from build123d import *

# Parameters (mm, degrees)
BOSS_EXTRUDE1_DEPTH = 165
SKETCH2_R           = 2.5
CUT_EXTRUDE1_DEPTH  = 167.021082999
SKETCH3_R           = 2.5
CUT_EXTRUDE2_DEPTH  = 167.021082999


with BuildPart() as part:
    # Sketch1 → Boss-Extrude1 (new, symmetric)
    with BuildSketch(Plane(origin=(0, 0, 0), x_dir=(0, 0, -1), z_dir=(1, 0, 0))):
        Polygon((11, 13), (13, 13), (13, -13), (-13, -13), (-13, -11), (11, -11), align=None)
    extrude(amount=BOSS_EXTRUDE1_DEPTH, both=True)

    # Sketch2 → Cut-Extrude1 (cut, through all)
    with BuildSketch(Plane(origin=(0, 0, 0), x_dir=(1, 0, 0), z_dir=(0, 1, 0))):
        with Locations(Location((150, -1, 0), (0, 0, 270))):
            Circle(SKETCH2_R)
    cut_extrude1 = extrude(amount=-CUT_EXTRUDE1_DEPTH, mode=Mode.SUBTRACT)

    # Mirror1: Cut-Extrude1 across plane
    add(cut_extrude1.mirror(Plane(origin=(0, 0, 0), x_dir=(0, 0, 1), z_dir=(1, 0, 0))), mode=Mode.SUBTRACT)

    # Sketch3 → Cut-Extrude2 (cut, through all)
    with BuildSketch(Plane(origin=(0, 0, 0), x_dir=(1, 0, 0), z_dir=(0, 1, 0))):
        with Locations(Location((100, 0, 0), (0, 0, 270))):
            Circle(SKETCH3_R)
    cut_extrude2 = extrude(amount=-CUT_EXTRUDE2_DEPTH, mode=Mode.SUBTRACT)

    # Mirror2: Cut-Extrude2 across plane
    add(cut_extrude2.mirror(Plane(origin=(0, 0, 0), x_dir=(0, 0, 1), z_dir=(1, 0, 0))), mode=Mode.SUBTRACT)


solid = part.part
Check sheet for the modelled part. Datum: model origin and axes. Units: mm. A direction names the side the tool comes from. Give positions to 0.01 mm unless a question says otherwise; leave off trailing zeros. Write each loop counter-clockwise with the first axis right and the second up, starting at its lowest first coordinate (ties: lowest second). Pieces come first, ordered by that corner, then holes. Notation, with made-up numbers: (-24.75, -35.5) -> (28.25, -35.5) arc R20 ccw to (28.25, -25.5) -> close; hole circle Ø7 at (89.5, 79). An arc over 180 degrees is marked (long way). One line per item, written item: value. Start each with the question number.
Item 1: Draft check along Z on faces 3 (the flat face through (2, -11, 1)), 4 (the cylindrical face through (-152.48, -11.99, 0.67)), 5 (the flat face through (2, 0, -13)). Enter one of: +Z half, -Z half, draft (parallel to the pull), parting line (faces both ways), or undercut.
Item 2: Section check B-B on y = 0. Record the cut outline in (x, z), then the cut area to 3 significant figures.
Item 3: Material ranges on probe 1 along X at (y, z) = (-12.5, 1); probe 2 along X at (y, z) = (-11.7, 0); probe 3 along Z at (x, y) = (-150, -12.6), recorded low to high. Write a range as from..to.
Item 4: Section check A-A on x = 66.5. Record the cut outline in (y, z), then the cut area to 3 significant figures.
Item 5: Gauge pin test, flat ends, axial feed: pin 1 (8 mm diameter, centred on x = 85.5, y = 6, fed in from +Z); pin 2 (8 mm diameter, centred on x = 60, z = -2.5, fed in from +Y); pin 3 (4 mm diameter, centred on x = 150, z = 1, fed in from -Y); pin 4 (6.5 mm diameter, centred on x = -150, z = 1, fed in from -Y). Record the tip position at first contact, or that the pin passes through.
Item 6: Tool access check on faces 1 (the cylindrical face through (-102.48, -11.99, -0.33)), 2 (the flat face through (2, 1, -11)). Record the directions out of +Z, -Z, +X, -X, +Y, -Y that give a thin tool (end or side, any length) a straight path to the whole face; none if there is none.
Results list:
1. face 3: draft
1. face 4: undercut
1. face 5: -Z half
2. outline: (-165, -13) -> (165, -13) -> (165, -11) -> (-165, -11) -> close
2. area: 660 mm²
3. probe 1: -165..-152.5, -147.5..-102.29, -97.71..97.71, 102.29..147.5, 152.5..165
3. probe 2: -165..-152.29, -147.71..-102.5, -97.5..97.5, 102.5..147.71, 152.29..165
3. probe 3: -13..-1.5, 3.5..13
4. outline: (-13, -13) -> (13, -13) -> (13, -11) -> (-11, -11) -> (-11, 13) -> (-13, 13) -> close
4. area: 100 mm²
5. pin 1: z = -11
5. pin 2: y = -11
5. pin 3: through
5. pin 4: y = -13
6. face 1: +Y, -Y
6. face 2: +Z, +X, -X, +Y
